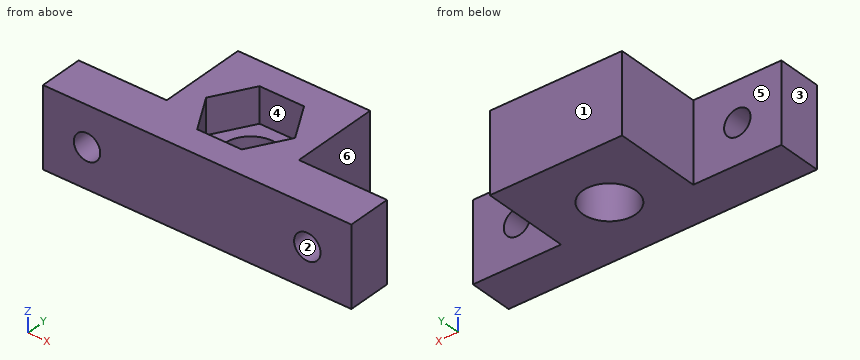
```python
from build123d import *

# Parameters (mm, degrees)
F0_R     = 6
F1_DEPTH = 18
F2_R     = 6
F3_DEPTH = 8
F4_R     = 3
F5_DEPTH = 25


with BuildPart() as f1:
    # F0 (on Top) → F1 (new body)
    with BuildSketch(Plane.XY):
        Polygon((0, 10), (0, 0), (70, 0), (70, 10), (50, 10), (50, 30), (20, 30), (20, 10), align=None)
        with Locations((35, 15)):
            Circle(F0_R, mode=Mode.SUBTRACT)
    extrude(amount=F1_DEPTH)

    # F2 (on face) → F3 (cut)
    with BuildSketch(Plane.XY.offset(18)):
        Polygon((40.051815, 23.75), (29.948185, 23.75), (24.89637, 15), (29.948185, 6.25), (40.051815, 6.25), (45.10363, 15), align=None)
        with Locations((35, 15)):
            Circle(F2_R, mode=Mode.SUBTRACT)
    extrude(amount=-F3_DEPTH, mode=Mode.SUBTRACT)

    # F4 (on face) → F5 (cut)
    with BuildSketch(Plane(origin=(0, 10, 0), x_dir=(-1, 0, 0), z_dir=(0, 1, 0))):
        with Locations((-60, 9)):
            Circle(F4_R)
        with Locations((-10, 9)):
            Circle(F4_R)
    extrude(amount=-F5_DEPTH, mode=Mode.SUBTRACT)


solid = f1.part
```
Source: CAD feature listing. Evaluate the final solid. Frame: model axes, mm. Face numbers are marked on the shaded views. A direction names the side the tool comes from. Give positions to 0.01 mm unless a question says otherwise; leave off trailing zeros. Write each loop counter-clockwise with the first axis right and the second up, starting at its lowest first coordinate (ties: lowest second). Pieces come first, ordered by that corner, then holes.
1. First-contact query: pin 1 (3.5 mm diameter, centred on x = 10, z = 9, fed in from +Y); pin 2 (9 mm diameter, centred on y = 24, z = 12, fed in from +X); pin 3 (4 mm diameter, centred on x = 58.5, z = 9, fed in from +Y); pin 4 (8 mm diameter, centred on y = 24, z = 11, fed in from -X). Flat tips, straight axial feed; report the tip coordinate or a pass-through.
2. Section query D-D (y = 19). Return the cut outline in (x, z), then the cut area to 3 significant figures.
3. Material intervals for line 1 along Y through (x, z) = (35, 2.25); line 2 along X through (y, z) = (4.5, 8); line 3 along X through (y, z) = (4.75, 10.5), sorted ascending.
4. Section query A-A (x = 60). Return the cut outline in (y, z).
5. Access query for the marked faces 4, 5 and 6. Directions: +Z, -Z, +X, -X, +Y, -Y. A direction counts if a zero-diameter tool reaches every point of the face in a straight line with its end or side. Return the directions, or none.
6. Section query B-B (z = 7). Return the cut outline in (x, y).
7. Section query C-C (y = 3.25). Return the cut outline in (x, z), then the cut area to 3 significant figures.
8. Pull-direction query (X, two-part tool) for the marked faces 1, 2 and 3; classes: +X half, -X half, draft (parallel to the pull), parting line (faces both ways), or undercut.
Output values:
1. pin 1: passes through
1. pin 2: stops at x = 50
1. pin 3: stops at y = 10
1. pin 4: stops at x = 20
2. outline: (20, 0) - (30.53, 0) - (30.53, 10) - (27.21, 10) - (27.21, 18) - (20, 18) - close; (39.47, 0) - (50, 0) - (50, 18) - (42.79, 18) - (42.79, 10) - (39.47, 10) - close
2. area: 326 mm2
3. line 1: y = 0 to 9, 21 to 30
3. line 2: x = 0 to 7.17, 12.83 to 57.17, 62.83 to 70
3. line 3: x = 0 to 7.4, 12.6 to 57.4, 62.6 to 70
4. outline: (0, 0) - (10, 0) - (10, 6) - (0, 6) - close; (0, 12) - (10, 12) - (10, 18) - (0, 18) - close
5. face 4: +Z
5. face 5: +Z, -Z, -X, +Y
5. face 6: +Z, -Z, +X, +Y
6. outline: (0, 0) - (7.76, 0) - (7.76, 10) - (0, 10) - close; (12.24, 0) - (57.76, 0) - (57.76, 10) - (50, 10) - (50, 30) - (20, 30) - (20, 10) - (12.24, 10) - close; (62.24, 0) - (70, 0) - (70, 10) - (62.24, 10) - close; hole circle Ø12 at (35, 15)
7. outline: (0, 0) - (70, 0) - (70, 18) - (0, 18) - close; hole circle Ø6 at (10, 9); hole circle Ø6 at (60, 9)
7. area: 1,200 mm2
8. face 1: draft
8. face 2: undercut
8. face 3: -X half
